Build history of the part. All positions in model axes, mm. A direction names the side the tool comes from. Round coordinates to 2 decimals unless told otherwise and drop trailing zeros. Write each loop counter-clockwise with the first axis right and the second up, starting at its lowest first coordinate (ties: lowest second). Pieces come first, ordered by that corner, then holes. Notation, with made-up numbers: (-26.5, -8) -> (1.5, -8) arc R17 ccw to (1.5, 10) -> close; hole circle Ø2 at (6.5, 41.5). An arc over 180 degrees is marked (long way). Answer in a Markdown table with one row per item. Add a question column.
from build123d import *

# Parameters (mm, degrees)
BOSS_EXTRUDE1_DEPTH = 4.445
SKETCH2_R           = 1.651
CUT_EXTRUDE1_DEPTH  = 108.429567879


with BuildPart() as part:
    # Sketch1 → Boss-Extrude1 (new body)
    with BuildSketch(Plane(origin=(0, 0, 0), x_dir=(1, 0, 0), z_dir=(0, 1, 0))):
        with BuildLine():
            Line((13.535585603, 0.635), (105.718351485, 0.635))
            Line((105.718351485, 0.635), (105.718351485, -14.9225))
            Line((105.718351485, -14.9225), (13.535585603, -14.9225))
            ThreePointArc((13.535585603, -14.9225), (12.61737712, -15.094274254), (11.823361218, -15.586363636))
            ThreePointArc((11.823361218, -15.586363636), (-7.311648515, -7.14375), (11.823361218, 1.298863636))
            ThreePointArc((11.823361218, 1.298863636), (12.61737712, 0.806774254), (13.535585603, 0.635))
        make_face()
        Polygon((0, 0), (8.23670297, 0), (12.373351485, -7.14375), (8.23670297, -14.2875), (0, -14.2875), (-4.136648515, -7.14375), align=None, mode=Mode.SUBTRACT)
    extrude(amount=BOSS_EXTRUDE1_DEPTH)

    # Sketch2 → Cut-Extrude1 (cut, through all)
    with BuildSketch(Plane(origin=(0, 4.445, 0), x_dir=(1, 0, 0), z_dir=(0, 1, 0))):
        with Locations(Location((93.018351485, -7.14375, 0), (0, 0, 270))):
            Circle(SKETCH2_R)
        with Locations(Location((67.618351485, -7.14375, 0), (0, 0, 270))):
            Circle(SKETCH2_R)
    extrude(amount=-CUT_EXTRUDE1_DEPTH, mode=Mode.SUBTRACT)


solid = part.part
(1) Saw through at B-B (y = 3.65). List the corners of the cut face in (x, z) (1 decimal), plus the area to 3 significant figures.
(2) Which spindle directions (+Z, -Z, +X, -X, +Y, -Y) get a long thin tool onto all of the face, cutting with end or side? Do faces 5 (the face through (60, 2, 14.922)), 6 (the face through (10.276, 2.191, 3.522)), 7 (the face through (59, 2, -0.635)). Say none if no direction does.
(3) Drop flat-ended pins along their axis: P1, Ø1, axis at x = 7, y = 2.5, coming from the +Z side; P2, Ø2, axis at x = 24.5, y = 1.5, coming from the +Z side; P3, Ø1.3, axis at x = 5, y = 1, coming from the -Z side; P4, Ø2, axis at x = 67.62, z = 7.14, coming from the +Y side. Give the stop position or say it passes through.
(4) Saw through at A-A (z = 11). List the corners of the cut face in (x, y) (1 decimal), plus the area to 3 significant figures.
(5) Saw through at D-D (x = 17.5). List the corners of the cut face in (y, z) (1 decimal).
(6) Saw through at C-C (z = 3). List the corners of the cut face in (x, y) (3 decimals), plus the area to 3 significant figures.
(7) Mould opens along X. For faces 1 (the face through (66.154, 2.254, 7.906)), 2 (the face through (-2.097, 2.191, 3.622)), 3 (the face through (105.718, 2, 7)), 4 (the face through (-7.306, 2.191, 7.513)) say: pulls with the +X half, pulls with the -X half, needs draft (parallel to the pull), parting line crosses it, or undercut.
(8) Probe line 1 along Z through (x, y) = (3.5, 1.7); line 2 along Z through (x, y) = (57.5, 3.8) (1 decimal); line 3 along Z through (x, y) = (2, 2.7). List the from-to ranges inside material, lowest first.
Answer sheet:
| question | item | result |
|---|---|---|
| 1 | outline | (11.8, -1.3) arc R2.5 cw to (13.5, -0.6) -> (105.7, -0.6) -> (105.7, 14.9) -> (13.5, 14.9) arc R2.5 cw to (11.8, 15.6) arc R11.4 ccw (long way) to start; hole (-4.1, 7.1) -> (0, 0) -> (8.2, 0) -> (12.4, 7.1) -> (8.2, 14.3) -> (0, 14.3) -> close; hole circle Ø3.3 at (67.6, 7.1); hole circle Ø3.3 at (93, 7.1) |
| 1 | area | 1,630 mm² |
| 2 | face 5 | +Z, +X, +Y, -Y |
| 2 | face 6 | +Y, -Y |
| 2 | face 7 | -Z, +X, +Y, -Y |
| 3 | P1 | stops at z = 18.32 |
| 3 | P2 | stops at z = 14.92 |
| 3 | P3 | stops at z = -4.28 |
| 3 | P4 | passes through |
| 4 | outline | (-6.6, 0) -> (-1.9, 0) -> (-1.9, 4.4) -> (-6.6, 4.4) -> close; (10.1, 0) -> (105.7, 0) -> (105.7, 4.4) -> (10.1, 4.4) -> close |
| 4 | area | 446 mm² |
| 5 | outline | (0, -0.6) -> (4.4, -0.6) -> (4.4, 14.9) -> (0, 14.9) -> close |
| 6 | outline | (-6.534, 0) -> (-1.737, 0) -> (-1.737, 4.445) -> (-6.534, 4.445) -> close; (9.974, 0) -> (105.718, 0) -> (105.718, 4.445) -> (9.974, 4.445) -> close |
| 6 | area | 447 mm² |
| 7 | face 1 | undercut |
| 7 | face 2 | undercut |
| 7 | face 3 | pulls with the +X half |
| 7 | face 4 | parting line crosses it |
| 8 | line 1 | z = -4.27 to 0, 14.29 to 18.56 |
| 8 | line 2 | z = -0.6 to 14.9 |
| 8 | line 3 | z = -4.09 to 0, 14.29 to 18.38 |
